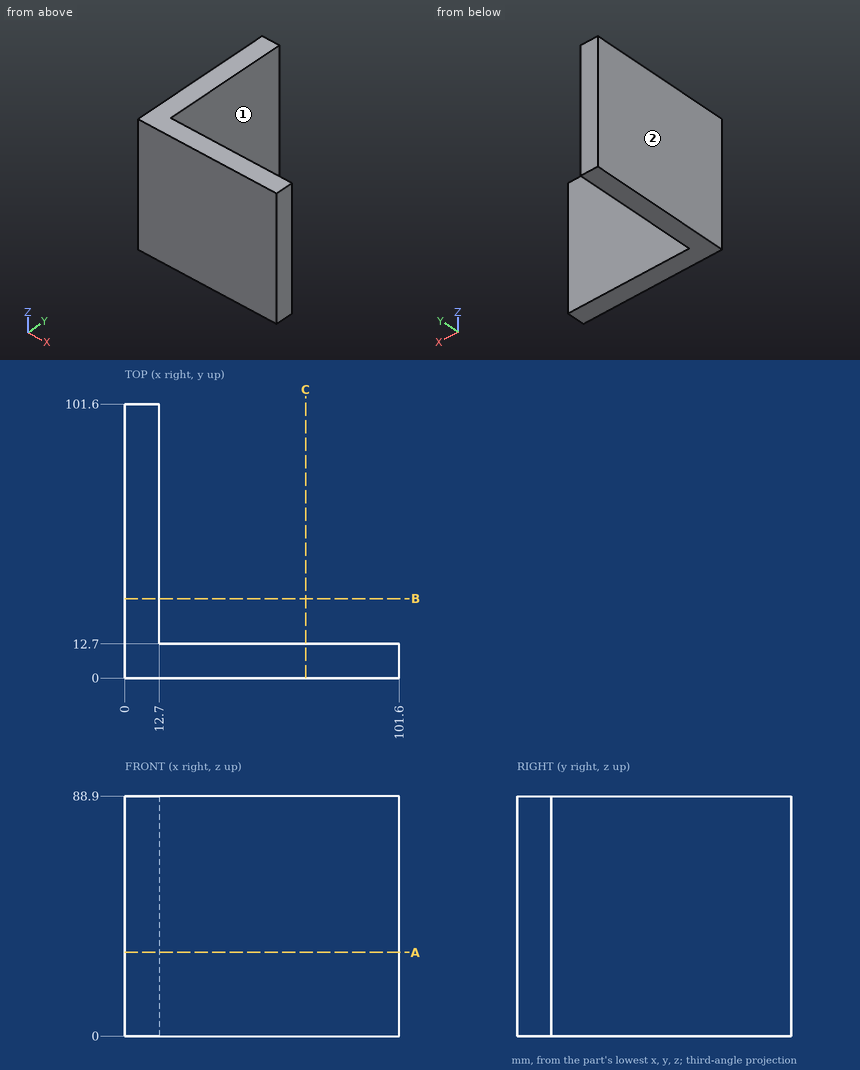
Answer from the drawing. Dimensions are ordinates in mm from the lowest x, y and z of the part. A direction names the side the tool comes from. Coordinates: 2 decimals unless noted, no trailing zeros. Write each loop counter-clockwise with the first axis right and the second up, starting at its lowest first coordinate (ties: lowest second). Pieces come first, ordered by that corner, then holes. Notation, with made-up numbers: (39, 27.5) - (69, 27.5) arc R15 ccw to (69, 52.5) - close; hole circle Ø4 at (74.5, 35). An arc over 180 degrees is marked (long way). Return JSON: item names as keys, results as strings. Group by question number.
Q1. Find the intervals of material crossed by line 1 along Y through (x, z) = (79, 21.5), in increasing order. Write a range as [from, to].
Q2. The part is cut by section B-B on y = 29.5. Write down the section's boundary in (x, z).
Q3. Which of the six approach directions +Z, -Z, +X, -X, +Y, -Y give full straight-line access (tool end or side, diameter ignored) to the marked faces 1 and 2?
Q4. Flat-ended cylindrical pins translate along their axes: pin 1 Ø12 at (x, y) = (11, 22.5) entering from -Z; pin 2 Ø10 at (y, z) = (23, 29) entering from +X. Find the tip coordinate at first contact, or state that the pin passes through.
Q5. The part is cut by section A-A on z = 31. Write down the section's boundary in (x, y).
Evaluation:
{
 "1": {"line 1": "y = [0, 12.7]"},
 "2": {"outline": "(0, 0) - (12.7, 0) - (12.7, 88.9) - (0, 88.9) - close"},
 "3": {"face 1": "+Z, -Z, +X, +Y", "face 2": "+Z, -Z, -X, +Y, -Y"},
 "4": {"pin 1": "stops at z = 0", "pin 2": "stops at x = 12.7"},
 "5": {"outline": "(0, 0) - (101.6, 0) - (101.6, 12.7) - (12.7, 12.7) - (12.7, 101.6) - (0, 101.6) - close"}
}
